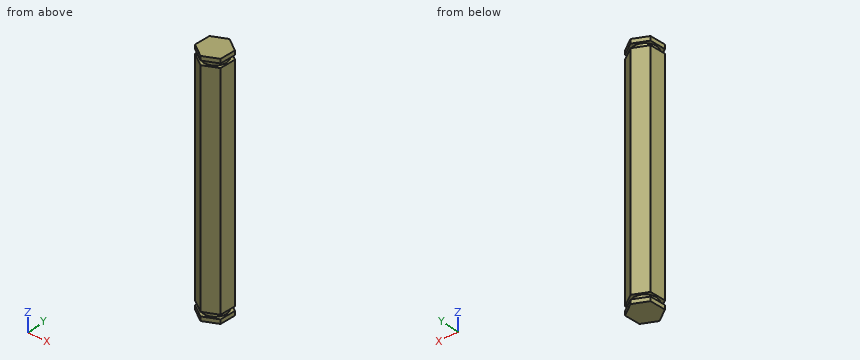
Solid Edge part; units mm, degrees
sketch "Sketch1" plane through (0, 0, 0) normal (0, 0, 1) x (1, 0, 0)
  line L0 (-6.1009, 4.0673) -> (-6.5728, -3.2499)
  line L1 (-6.5728, -3.2499) -> (-0.4719, -7.3171)
  line L2 (-0.4719, -7.3171) -> (6.1009, -4.0673)
  line L3 (6.1009, -4.0673) -> (6.5728, 3.2499)
  line L4 (6.5728, 3.2499) -> (0.4719, 7.3171)
  line L5 (0.4719, 7.3171) -> (-6.1009, 4.0673)
extrude "Protrusion1" add sketch "Sketch1" against normal blind 115
sketch "Sketch2" plane through (0, 0, -2) normal (0, 0, 1) x (-0.8964, -0.4432, 0)
  circle A0 centre (0, 0) radius 5.5
  circle A1 centre (0, 0) radius 13.1424
extrude "ExtrudedCutout_1" cut sketch "Sketch2" against normal blind 2
sketch "Sketch3" plane through (0, 0, -113) normal (0, 0, -1) x (0.8964, 0.4432, 0)
  circle A0 centre (0, 0) radius 5.5
  circle A1 centre (0, 0) radius 13.1424
extrude "ExtrudedCutout_2" cut sketch "Sketch3" against normal blind 2
properties part number "BumbleB0649"
Check sheet for the modelled part. Datum: model origin and axes. Units: mm. Coordinates: 2 decimals unless noted, no trailing zeros. Write each loop counter-clockwise with the first axis right and the second up, starting at its lowest first coordinate (ties: lowest second). Pieces come first, ordered by that corner, then holes.
Item 1: Cross-section at C-C on y = 0. Record the boundary of the cut face in (x, z), then the cut area to 3 significant figures.
Numbers:
outline: (-6.36, -115) - (6.36, -115) - (6.36, -113) - (5.5, -113) - (5.5, -111) - (6.36, -111) - (6.36, -4) - (5.5, -4) - (5.5, -2) - (6.36, -2) - (6.36, 0) - (-6.36, 0) - (-6.36, -2) - (-5.5, -2) - (-5.5, -4) - (-6.36, -4) - (-6.36, -111) - (-5.5, -111) - (-5.5, -113) - (-6.36, -113) - close
area: 1,460 mm2
Item 2: Cross-section at A-A on z = -68. Record the boundary of the cut face in (x, y).
Numbers:
outline: (-6.57, -3.25) - (-0.47, -7.32) - (6.1, -4.07) - (6.57, 3.25) - (0.47, 7.32) - (-6.1, 4.07) - close
Item 3: Cross-section at B-B on x = 2. Record the boundary of the cut face in (y, z), then the cut area to 3 significant figures.
Numbers:
outline: (-6.09, -115) - (6.3, -115) - (6.3, -113) - (5.12, -113) - (5.12, -111) - (6.3, -111) - (6.3, -4) - (5.12, -4) - (5.12, -2) - (6.3, -2) - (6.3, 0) - (-6.09, 0) - (-6.09, -2) - (-5.12, -2) - (-5.12, -4) - (-6.09, -4) - (-6.09, -111) - (-5.12, -111) - (-5.12, -113) - (-6.09, -113) - close
area: 1,420 mm2
Item 4: Depth check by flat-ended pin: pin 1 Ø6 at (x, z) = (-3.5, -55) entering from -Y; pin 2 Ø4 at (x, z) = (-3.5, -82.5) entering from -Y; pin 3 Ø1.5 at (y, z) = (-0.5, -68) entering from +X. Enter the tip coordinate at first touch or a pass-through.
Numbers:
pin 1: stops at y = -7.3
pin 2: stops at y = -6.63
pin 3: stops at x = 6.38
Item 5: Scan lines: probe 1 along Z at (x, y) = (-5, -3); probe 2 along Y at (x, z) = (-5, -86); probe 3 along Y at (x, z) = (-2.75, -85.5). Record each from-to range of solid material in increasing order.
Numbers:
probe 1: z = -115 to -113, -111 to -4, -2 to 0
probe 2: y = -4.3 to 4.61
probe 3: y = -5.8 to 5.72
